Source: CAD feature listing. Evaluate the final solid. Frame: model axes, mm. Face numbers are marked on the shaded views. Round coordinates to 2 decimals unless told otherwise and drop trailing zeros. Write each loop counter-clockwise with the first axis right and the second up, starting at its lowest first coordinate (ties: lowest second). Pieces come first, ordered by that corner, then holes. Notation, with made-up numbers: M 55.25,24 L 85.25,24 A9 cw 85.25,30 Z; hole C -5,-38.75 d4. An arc over 180 degrees is marked long. Use a Markdown table: item, result.
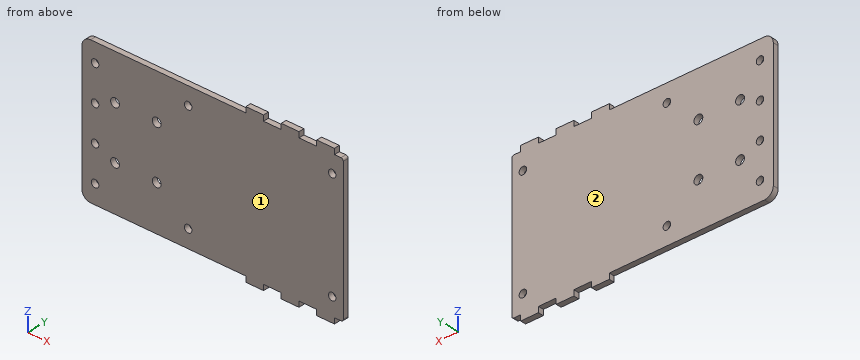
```python
from build123d import *

# Parameters (mm, degrees)
SKETCH1_W                     = 10.16
SKETCH1_H                     = 3.175
MAIN_EXTRUDE_DEPTH            = 3.175
SKETCH2_R                     = 2.54
CASTER_MOUNTING_HOLES_DEPTH   = 89.274136218
SKETCH3_W                     = 2.54
SKETCH3_H                     = 82.55
REMOVE_UNEVEN_BACK_EDGE_DEPTH = 89.274136218
SKETCH5_R                     = 2.15
STANDOFF_HOLES_DEPTH          = 89.274136218
FILLET1_R                     = 5.08
FILLET2_R                     = 1.27
FILLET3_R                     = 1.27
SKETCH9_R                     = 2.15
FRONT_MOUNTING_HOLES_DEPTH    = 89.274136218


with BuildPart() as part:
    # Sketch1 → Main Extrude (new body)
    with BuildSketch(Plane(origin=(0, 0, 0), x_dir=(1, 0, 0), z_dir=(0, 1, 0))):
        with Locations((22.86, -42.8625)):
            Rectangle(SKETCH1_W, SKETCH1_H)
        Polygon((27.94, -41.275), (38.1, -41.275), (48.26, -41.275), (58.42, -41.275), (68.58, -41.275), (76.2, -41.275), (76.2, 41.275), (68.58, 41.275), (58.42, 41.275), (48.26, 41.275), (38.1, 41.275), (27.94, 41.275), (17.78, 41.275), (-76.2, 41.275), (-76.2, -41.275), (17.78, -41.275), align=None)
        with Locations((43.18, -42.8625)):
            Rectangle(SKETCH1_W, SKETCH1_H)
        with Locations((22.86, 42.8625)):
            Rectangle(SKETCH1_W, SKETCH1_H)
        with Locations((63.5, -42.8625)):
            Rectangle(SKETCH1_W, SKETCH1_H)
        with Locations((63.5, 42.8625)):
            Rectangle(SKETCH1_W, SKETCH1_H)
        with Locations((43.18, 42.8625)):
            Rectangle(SKETCH1_W, SKETCH1_H)
    extrude(amount=MAIN_EXTRUDE_DEPTH)

    # Sketch2 → Caster Mounting Holes (cut, through all)
    with BuildSketch(Plane(origin=(0, 3.175, 0), x_dir=(1, 0, 0), z_dir=(0, 1, 0))):
        with Locations(Location((-57.15, 15.24, 0), (0, 0, 270))):
            Circle(SKETCH2_R)
        with Locations(Location((-33.274, 15.24, 0), (0, 0, 270))):
            Circle(SKETCH2_R)
        with Locations(Location((-33.274, -15.24, 0), (0, 0, 270))):
            Circle(SKETCH2_R)
        with Locations(Location((-57.15, -15.24, 0), (0, 0, 270))):
            Circle(SKETCH2_R)
    extrude(amount=-CASTER_MOUNTING_HOLES_DEPTH, mode=Mode.SUBTRACT)

    # Sketch3 → Remove Uneven Back Edge (cut, through all)
    with BuildSketch(Plane(origin=(0, 3.175, 0), x_dir=(1, 0, 0), z_dir=(0, 1, 0))):
        with Locations((74.93, 0)):
            Rectangle(SKETCH3_W, SKETCH3_H)
    extrude(amount=-REMOVE_UNEVEN_BACK_EDGE_DEPTH, mode=Mode.SUBTRACT)

    # Sketch5 → Standoff Holes (cut, through all)
    with BuildSketch(Plane(origin=(0, 3.175, 0), x_dir=(1, 0, 0), z_dir=(0, 1, 0))):
        with Locations(Location((-15.24, 31.115, 0), (0, 0, 270))):
            Circle(SKETCH5_R)
        with Locations(Location((67.31, 31.115, 0), (0, 0, 270))):
            Circle(SKETCH5_R)
        with Locations(Location((67.31, -31.115, 0), (0, 0, 270))):
            Circle(SKETCH5_R)
        with Locations(Location((-15.24, -31.115, 0), (0, 0, 270))):
            Circle(SKETCH5_R)
    extrude(amount=-STANDOFF_HOLES_DEPTH, mode=Mode.SUBTRACT)

    # Fillet1
    fillet1_edges = [part.edges().sort_by_distance(p)[0] for p in [
        (-76.2, 1.5875, 41.275),
        (-76.2, 1.5875, -41.275),
    ]]
    fillet(fillet1_edges, radius=FILLET1_R)

    # Fillet2
    fillet2_edges = [part.edges().sort_by_distance(p)[0] for p in [
        (73.66, 1.5875, 41.275),
    ]]
    fillet(fillet2_edges, radius=FILLET2_R)

    # Fillet3
    fillet3_edges = [part.edges().sort_by_distance(p)[0] for p in [
        (73.66, 1.5875, -41.275),
    ]]
    fillet(fillet3_edges, radius=FILLET3_R)

    # Sketch9 → Front Mounting Holes (cut, through all)
    with BuildSketch(Plane(origin=(0, 3.175, 0), x_dir=(1, 0, 0), z_dir=(0, 1, 0))):
        with Locations(Location((-68.58, -30.48, 0), (0, 0, 270))):
            Circle(SKETCH9_R)
        with Locations(Location((-68.58, -10.16, 0), (0, 0, 270))):
            Circle(SKETCH9_R)
        with Locations(Location((-68.58, 10.16, 0), (0, 0, 270))):
            Circle(SKETCH9_R)
        with Locations(Location((-68.58, 30.48, 0), (0, 0, 270))):
            Circle(SKETCH9_R)
    extrude(amount=-FRONT_MOUNTING_HOLES_DEPTH, mode=Mode.SUBTRACT)


solid = part.part
```
Q1. First-contact query: pin 1 Ø1 at (x, y) = (70, 2) entering from -Z (3 decimals); pin 2 Ø4 at (x, z) = (-68.58, 30.48) entering from +Y; pin 3 Ø1.6 at (y, z) = (1, 43) entering from -X; pin 4 Ø5.5 at (x, z) = (-15.24, 31.115) entering from +Y (3 decimals). Flat tips, straight axial feed; report the tip coordinate or a pass-through.
Results are:
| item | result |
|---|---|
| pin 1 | z = -41.275 |
| pin 2 | through |
| pin 3 | x = 17.78 |
| pin 4 | y = 3.175 |
Q2. Mould query, pull axis Y, two halves, no side actions, for the marked faces 1 and 2. Classes: +Y half, -Y half, draft (parallel to the pull), parting line (faces both ways), or undercut.
Results are:
| item | result |
|---|---|
| face 1 | -Y half |
| face 2 | +Y half |
Q3. Line query: L1, parallel to X at y = 1.8, z = -15.24; L2, parallel to Z at x = -55, y = 1.65 (3 decimals); L3, parallel to X at y = 2.2, z = 14. Output: solid intervals per line, ascending.
Results are:
| item | result |
|---|---|
| L1 | -76.2 to -59.69, -54.61 to -35.81, -30.73 to 73.66 |
| L2 | -41.275 to -16.592, -13.888 to 13.888, 16.592 to 41.275 |
| L3 | -76.2 to -59.37, -54.93 to -35.49, -31.06 to 73.66 |
Q4. Section B-B on z = -10.16. Return loops of the section in (x, y) (3 decimals), plus the area to 3 significant figures.
Results are:
| item | result |
|---|---|
| outline | M -76.2,0 L -70.73,0 L -70.73,3.175 L -76.2,3.175 Z; M -66.43,0 L 73.66,0 L 73.66,3.175 L -66.43,3.175 Z |
| area | 462 mm^2 |
Q5. Section A-A on x = -15.24. Return loops of the section in (y, z) (3 decimals), plus the area to 3 significant figures.
Results are:
| item | result |
|---|---|
| outline | M 0,-41.275 L 3.175,-41.275 L 3.175,-33.265 L 0,-33.265 Z; M 0,-28.965 L 3.175,-28.965 L 3.175,28.965 L 0,28.965 Z; M 0,33.265 L 3.175,33.265 L 3.175,41.275 L 0,41.275 Z |
| area | 235 mm^2 |
Q6. Section C-C on x = -68.58. Return loops of the section in (y, z) (3 decimals).
Results are:
| item | result |
|---|---|
| outline | M 0,-41.275 L 3.175,-41.275 L 3.175,-32.63 L 0,-32.63 Z; M 0,-28.33 L 3.175,-28.33 L 3.175,-12.31 L 0,-12.31 Z; M 0,-8.01 L 3.175,-8.01 L 3.175,8.01 L 0,8.01 Z; M 0,12.31 L 3.175,12.31 L 3.175,28.33 L 0,28.33 Z; M 0,32.63 L 3.175,32.63 L 3.175,41.275 L 0,41.275 Z |
Q7. Section D-D on y = 2. Give the number of separate pieces and of enclosed holes in the cut face, plus the area to 3 significant figures.
Results are:
| item | result |
|---|---|
| separate pieces | 1 |
| enclosed holes | 12 |
| area | 12,400 mm^2 |
